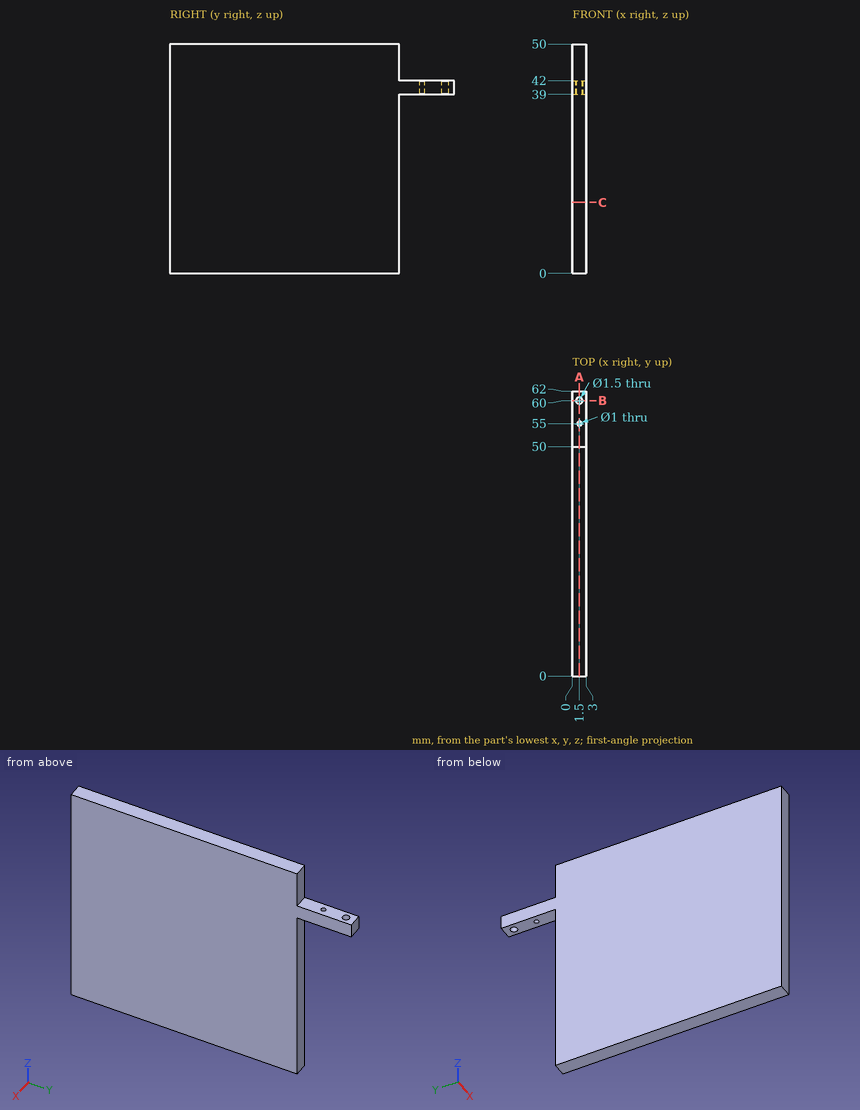
Check sheet for the drawn part. Datum: minimum x, y, z corner. Units: mm. Coordinates: 2 decimals unless noted, no trailing zeros. Loops run counter-clockwise (first coordinate to the right, second up) from the corner with the lowest first, then second, coordinate; pieces in that order, holes last. Notation, with made-up numbers: (-36.5, 44) -> (-32.5, 44) arc R19 ccw to (-32.5, 78) -> close; hole circle Ø7 at (39, 5.5). An arc over 180 degrees is marked (long way). Answer in a Markdown table with one row per item.
1) Depth check by flat-ended pin: P1, Ø0.9, axis at x = 2, y = 54, coming from the +Z side; P2, Ø0.9, axis at x = 1.5, y = 60, coming from the +Z side. Enter the tip coordinate at first touch or a pass-through.
The answers:
| item | result |
|---|---|
| P1 | stops at z = 42 |
| P2 | passes through |
2) Scan lines: line 1 along Y through (x, z) = (1.5, 40.75); line 2 along X through (y, z) = (60, 39.7); line 3 along X through (y, z) = (55, 40). Record each from-to range of solid material in increasing order. Write a range as from..to.
The answers:
| item | result |
|---|---|
| line 1 | y = 0..54.5, 55.5..59.25, 60.75..62 |
| line 2 | x = 0..0.75, 2.25..3 |
| line 3 | x = 0..1, 2..3 |
3) Section check A-A (x = 1.5). Record the cut outline in (y, z), and give its area (3 significant figures).
The answers:
| item | result |
|---|---|
| outline | (0, 0) -> (50, 0) -> (50, 39) -> (54.5, 39) -> (54.5, 42) -> (50, 42) -> (50, 50) -> (0, 50) -> close; (55.5, 39) -> (59.25, 39) -> (59.25, 42) -> (55.5, 42) -> close; (60.75, 39) -> (62, 39) -> (62, 42) -> (60.75, 42) -> close |
| area | 2,530 mm2 |
4) Section check B-B (y = 60). Record the cut outline in (x, z), and give its area (3 significant figures).
The answers:
| item | result |
|---|---|
| outline | (0, 39) -> (0.75, 39) -> (0.75, 42) -> (0, 42) -> close; (2.25, 39) -> (3, 39) -> (3, 42) -> (2.25, 42) -> close |
| area | 4.50 mm2 |
5) Section check C-C (z = 15.5). Record the cut outline in (x, y), and give its area (3 significant figures).
The answers:
| item | result |
|---|---|
| outline | (0, 0) -> (3, 0) -> (3, 50) -> (0, 50) -> close |
| area | 150 mm2 |
